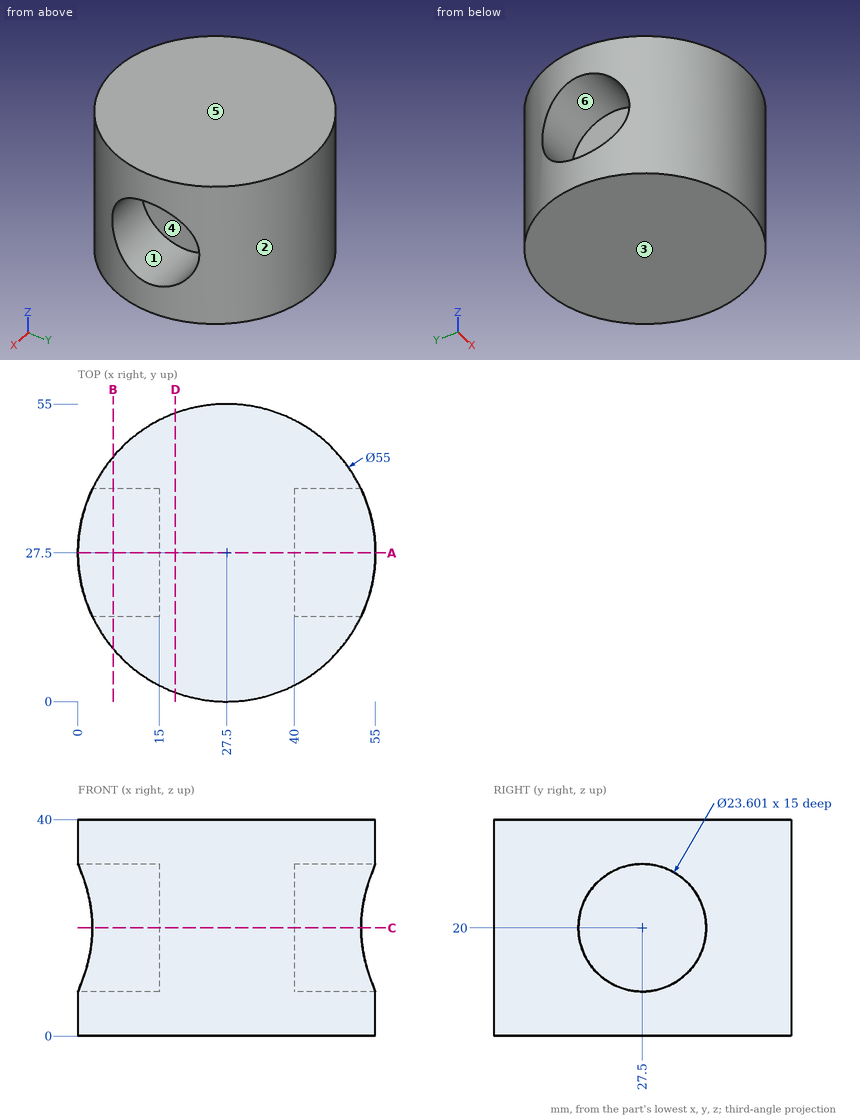
Job drawing, mm, ordinate dimensions from the low corner. One solid piece. A direction names the side the tool comes from. Round coordinates to 2 decimals unless told otherwise and drop trailing zeros. Write each loop counter-clockwise with the first axis right and the second up, starting at its lowest first coordinate (ties: lowest second). Pieces come first, ordered by that corner, then holes. Notation, with made-up numbers: (77.5, 78) -> (109.5, 78) arc R22 cw to (109.5, 106) -> close; hole circle Ø7 at (58, -17). An arc over 180 degrees is marked (long way). Answer as a JSON object with one key per item and string values.
(1) Band-saw the part on C-C, the plane z = 20. List the corners of the cut face in (x, y), then the cut area to 3 significant figures.
Reported:
{"outline": "(2.66, 15.7) arc R27.5 ccw to (52.34, 15.7) -> (40, 15.7) -> (40, 39.3) -> (52.34, 39.3) arc R27.5 ccw to (2.66, 39.3) -> (15, 39.3) -> (15, 15.7) -> close", "area": "1,710 mm^2"}
(2) Which spindle directions (+Z, -Z, +X, -X, +Y, -Y) get a long thin tool onto all of the face, cutting with end or side? Do the marked faces 4, 5 and 6. Say none if no direction does.
Reported:
{"face 4": "+X", "face 5": "+Z, +X, -X, +Y, -Y", "face 6": "-X"}
(3) Pin check, flat tips, straight feed: P1, Ø14, axis at y = 27.5, z = 20, coming from the -X side; P2, Ø2, axis at y = 42, z = 22, coming from the -X side; P3, Ø8, axis at y = 37, z = 28.5, coming from the +X side. Stop position of each tip, or through.
Reported:
{"P1": "stops at x = 15", "P2": "stops at x = 3.54", "P3": "stops at x = 54.36"}
(4) Band-saw the part on D-D, the plane x = 18. List the corners of the cut face in (y, z), then the cut area to 3 significant figures.
Reported:
{"outline": "(1.69, 0) -> (53.31, 0) -> (53.31, 40) -> (1.69, 40) -> close", "area": "2,060 mm^2"}
(5) Band-saw the part on A-A, the plane y = 27.5. List the corners of the cut face in (x, z).
Reported:
{"outline": "(0, 0) -> (55, 0) -> (55, 8.2) -> (40, 8.2) -> (40, 31.8) -> (55, 31.8) -> (55, 40) -> (0, 40) -> (0, 31.8) -> (15, 31.8) -> (15, 8.2) -> (0, 8.2) -> close"}
(6) Two-plate mould, pull along Y, no slides. Class the marked faces 1, 2 and 3: +Y half, -Y half, draft (parallel to the pull), parting line (faces both ways), or undercut.
Reported:
{"face 1": "undercut", "face 2": "parting line", "face 3": "draft"}
(7) Probe probe 1 along Z at (x, y) = (7, 27); probe 2 along X at (y, z) = (34, 18); probe 3 along Y at (x, z) = (27.5, 22). List the from-to ranges inside material, lowest first. Write a range as [from, to].
Reported:
{"probe 1": "z = [0, 8.21], [31.79, 40]", "probe 2": "x = [15, 40]", "probe 3": "y = [0, 55]"}
(8) Band-saw the part on B-B, the plane x = 6.5. List the corners of the cut face in (y, z).
Reported:
{"outline": "(9.74, 0) -> (45.26, 0) -> (45.26, 40) -> (9.74, 40) -> close; hole circle Ø23.6 at (27.5, 20)"}
